Part model, mm, in its own coordinate system. Coordinates: 2 decimals unless noted, no trailing zeros. Order: outer loops, then holes, each group sorted by start corner. A loop starts at its lowest first (then second) coordinate and runs counter-clockwise, first axis right, second up.
1) Cut at B-B (x = 0). List the corners of the cut face in (y, z) (3 decimals), and give its area (3 significant figures).
2) Mould opens along Y. For faces 1 (the flat face through (-1, 1, 3.175)), 2 (the cylindrical face through (51.873, 68.68, 1.565)), 3 (the flat face through (1, -76.2, 2)) say: +Y half, -Y half, draft (parallel to the pull), parting line (faces both ways), or undercut.
3) Cut at C-C (x = -50.8). List the corners of the cut face in (y, z) (1 decimal).
4) Wall check: L1, parallel to X at y = 69.85, z = 1.5; L2, parallel to Y at x = 0.5, z = 1.95; L3, parallel to X at y = -57.15, z = 1.8. Give the ranges that are in metal, low to high.
5) Cut at A-A (y = -57.15). List the corners of the cut face in (x, z) (3 decimals), and give its area (3 significant figures).
Autodesk Inventor part; units mm, degrees
ref_plane "YZ Plane" through (0, 0, 0) normal (1, 0, 0) x (0, 1, 0)
ref_plane "XZ Plane" through (0, 0, 0) normal (0, 1, 0) x (-1, 0, 0)
ref_plane "XY Plane" through (0, 0, 0) normal (0, 0, 1) x (1, 0, 0)
sketch "Sketch1" plane through (0, 0, 0) normal (0, 0, 1) x (1, 0, 0)
  line L0 (0, 0) -> (0, 40.5449) construction
  line L1 (0, 0) -> (42.3786, 0) construction
  line L2 (-57.15, 76.2) -> (57.15, 76.2)
  line L3 (57.15, 76.2) -> (57.15, -76.2)
  line L4 (57.15, -76.2) -> (-57.15, -76.2)
  line L5 (-57.15, -76.2) -> (-57.15, 76.2)
  dimension "d0" = 152.4
  dimension "d1" = 114.3
extrude "Extrusion1" add sketch "Sketch1" along normal blind 3.175
sketch "Sketch2" plane through (0, 0, 3.175) normal (0, 0, 1) x (1, 0, 0)
  line L0 (-57.15, 76.2) -> (-57.15, -76.2)
  line L1 (-57.15, -76.2) -> (57.15, -76.2)
  point P0 (0, 0)
  point P1 (0, -57.15)
  dimension "d5" = 57.15
  dimension "d22" = 19.05
hole "Hole1" at (0, -57.15, 3.175) direction (0, 0, -1) diameter 12.7 end through all
sketch "Sketch3" plane through (0, 0, 3.175) normal (0, 0, 1) x (1, 0, 0)
  line L0 (-57.15, -76.2) -> (57.15, -76.2)
  line L1 (-57.15, 76.2) -> (-57.15, -76.2)
  point P0 (0, 0)
  point P1 (-50.8, -69.85)
  dimension "d13" = 6.35
  dimension "d14" = 6.35
hole "Hole2" at (-50.8, -69.85, 3.175) direction (0, 0, -1) diameter 3.175 end through all
mirror "Mirror1" about plane through (0, 0, 0) normal (1, 0, 0) of "Hole2"
mirror "Mirror2" about plane through (0, 0, 0) normal (0, 1, 0) of "Hole2", "Mirror1"
properties part number "GearBoxFrontPlate"
Geometry check:
1. outline: (-76.2, 0) - (-63.5, 0) - (-63.5, 3.175) - (-76.2, 3.175) - close; (-50.8, 0) - (76.2, 0) - (76.2, 3.175) - (-50.8, 3.175) - close
1. area: 444 mm2
2. face 1: draft
2. face 2: undercut
2. face 3: -Y half
3. outline: (-76.2, 0) - (-71.4, 0) - (-71.4, 3.2) - (-76.2, 3.2) - close; (-68.3, 0) - (68.3, 0) - (68.3, 3.2) - (-68.3, 3.2) - close; (71.4, 0) - (76.2, 0) - (76.2, 3.2) - (71.4, 3.2) - close
4. L1: x = -57.15 to -52.39, -49.21 to 49.21, 52.39 to 57.15
4. L2: y = -76.2 to -63.48, -50.82 to 76.2
4. L3: x = -57.15 to -6.35, 6.35 to 57.15
5. outline: (-57.15, 0) - (-6.35, 0) - (-6.35, 3.175) - (-57.15, 3.175) - close; (6.35, 0) - (57.15, 0) - (57.15, 3.175) - (6.35, 3.175) - close
5. area: 323 mm2
